Here's how the part is built. I have some questions about the finished solid (model axes, mm). A direction names the side the tool comes from. Round coordinates to 2 decimals unless told otherwise and drop trailing zeros. Order: outer loops, then holes, each group sorted by start corner. A loop starts at its lowest first (then second) coordinate and runs counter-clockwise, first axis right, second up. Notation, with made-up numbers: M 16.25,53 L 43.25,53 A19 ccw 43.25,83 Z; hole C 47.25,60 d9. An arc over 180 degrees is marked long. Write item = value, one per line. Start each with the question number.
Item 1: For faces 1 (the face through (0, 0, 12)), 2 (the face through (1.3, -1.3, 10)), which set-ups out of +Z, -Z, +X, -X, +Y, -Y let a thin tool reach every point of the face, with its end or its side?
Item 2: Please list where these lines run through material, in increasing order: L1, parallel to X at y = 0.5, z = 6.25; L2, parallel to Y at x = 1.25, z = 7.75; L3, parallel to Z at x = -2.5, y = 1.25.
Item 3: I'm going to push flat-ended pins straight in: P1, Ø1, axis at y = -1.5, z = 2, coming from the -X side; P2, Ø1, axis at x = 0.5, y = -1.5, coming from the -Z side. Where does each tip first touch, or does it pass through?
Item 4: I want a section at A-A, the plane z = 7.5. List the corners of the cut face in (x, y) for me, plus the area to 3 significant figures.
Autodesk Inventor part; units mm, degrees
ref_plane "YZ Plane" through (0, 0, 0) normal (1, 0, 0) x (0, 1, 0)
ref_plane "XZ Plane" through (0, 0, 0) normal (0, 1, 0) x (-1, 0, 0)
ref_plane "XY Plane" through (0, 0, 0) normal (0, 0, 1) x (1, 0, 0)
sketch "スケッチ1" plane through (0, 0, 0) normal (0, 0, 1) x (1, 0, 0)
  circle A0 centre (0, 0) radius 1.5
  dimension "d0" = 3
extrude "押し出し1" add sketch "スケッチ1" along normal blind 10
sketch "スケッチ2" plane through (0, 0, 10) normal (0, 0, 1) x (1, 0, 0)
  circle A0 centre (0, 0) radius 1.5
  circle A1 centre (0, 0) radius 3
  dimension "d3" = 6
extrude "押し出し2" add sketch "スケッチ2" along normal blind 2 contours A0 | A1
fillet "フィレット1" radius 2 1 edges at (-3, 0, 12)
properties part number "M3ボタンボルト10" material "鋼、高強度、低合金"
Filled in:
q1.face_1 = +Z, +X, -X, +Y, -Y
q1.face_2 = -Z
q2.L1 = -1.41 to 1.41
q2.L2 = -0.83 to 0.83
q2.L3 = 10 to 10.88
q3.P1 = -1.12
q3.P2 = 0
q4.outline = C 0,0 d3
q4.area = 7.07 mm^2
